CAD build for the part. Positions are in the model's coordinates, mm. A direction names the side the tool comes from. Round coordinates to 2 decimals unless told otherwise and drop trailing zeros. Loops run counter-clockwise (first coordinate to the right, second up) from the corner with the lowest first, then second, coordinate; pieces in that order, holes last. Notation, with made-up numbers: M 29.25,6.5 L 72.25,6.5 A16 ccw 72.25,14.5 Z; hole C 66.5,87 d11. An arc over 180 degrees is marked long. Put each result on its own line as item: value. Start each with the question number.
from build123d import *

# Parameters (mm, degrees)
SKETCH1_W           = 25
SKETCH1_H           = 32
BOSS_EXTRUDE1_DEPTH = 2
SKETCH2_W           = 29
SKETCH2_H           = 36
SKETCH2_W_2         = 25
SKETCH2_H_2         = 32
BOSS_EXTRUDE2_DEPTH = 17
SKETCH3_W           = 18
SKETCH3_H           = 2
CUT_EXTRUDE1_DEPTH  = 2.7
SKETCH4_W           = 8
SKETCH4_H           = 2
CUT_EXTRUDE2_DEPTH  = 1.5
SKETCH7_W           = 1
SKETCH7_H           = 32
BOSS_EXTRUDE3_DEPTH = 15
SKETCH8_W           = 3
SKETCH8_H           = 7.46
CUT_EXTRUDE4_DEPTH  = 6
SKETCH9_W           = 3
SKETCH9_H           = 7.46
CUT_EXTRUDE5_DEPTH  = 6.5
SKETCH10_W          = 29
SKETCH10_H          = 3
BOSS_EXTRUDE4_DEPTH = 5
SKETCH11_W          = 29
SKETCH11_H          = 3
BOSS_EXTRUDE5_DEPTH = 5
SKETCH12_R          = 0.775
CUT_EXTRUDE6_DEPTH  = 4
FILLET1_R           = 5
SKETCH13_R          = 1.275
CUT_EXTRUDE7_DEPTH  = 1
SKETCH14_W          = 5
SKETCH14_H          = 3
BOSS_EXTRUDE6_DEPTH = 5
SKETCH15_W          = 5
SKETCH15_H          = 3
BOSS_EXTRUDE7_DEPTH = 5
SKETCH16_R          = 0.775
CUT_EXTRUDE8_DEPTH  = 5
FILLET2_R           = 2
SKETCH17_R          = 1.275
CUT_EXTRUDE9_DEPTH  = 1
SKETCH18_W          = 1.5
SKETCH18_H          = 5
CUT_EXTRUDE10_DEPTH = 42
SKETCH19_W          = 3
SKETCH19_H          = 3
CUT_EXTRUDE11_DEPTH = 18
SKETCH21_W          = 1.5
SKETCH21_H          = 5
CUT_EXTRUDE12_DEPTH = 2


with BuildPart() as part:
    # Sketch1 → Boss-Extrude1 (new body)
    with BuildSketch(Plane(origin=(0, 0, 0), x_dir=(1, 0, 0), z_dir=(0, 1, 0))):
        with Locations((-1.021545319, 9.369242199)):
            Rectangle(SKETCH1_W, SKETCH1_H)
    extrude(amount=BOSS_EXTRUDE1_DEPTH)

    # Sketch2 → Boss-Extrude2 (add)
    with BuildSketch(Plane(origin=(0, 2, 0), x_dir=(1, 0, 0), z_dir=(0, 1, 0))):
        with Locations((-1.021545319, 9.369242199)):
            Rectangle(SKETCH2_W, SKETCH2_H)
        with Locations((-1.021545319, 9.369242199)):
            Rectangle(SKETCH2_W_2, SKETCH2_H_2, mode=Mode.SUBTRACT)
    extrude(amount=-BOSS_EXTRUDE2_DEPTH)

    # Sketch3 → Cut-Extrude1 (cut)
    with BuildSketch(Plane.XZ.offset(15)):
        with Locations((-4.521545319, -26.369242199)):
            Rectangle(SKETCH3_W, SKETCH3_H)
    extrude(amount=-CUT_EXTRUDE1_DEPTH, mode=Mode.SUBTRACT)

    # Sketch4 → Cut-Extrude2 (cut)
    with BuildSketch(Plane.XZ.offset(15)):
        with Locations((-4.521545319, 7.630757801)):
            Rectangle(SKETCH4_W, SKETCH4_H)
    extrude(amount=-CUT_EXTRUDE2_DEPTH, mode=Mode.SUBTRACT)

    # Sketch7 → Boss-Extrude3 (add)
    with BuildSketch(Plane.XZ):
        with Locations((10.978454681, -9.369242199)):
            Rectangle(SKETCH7_W, SKETCH7_H)
    extrude(amount=BOSS_EXTRUDE3_DEPTH)

    # Sketch8 → Cut-Extrude4 (cut)
    with BuildSketch(Plane.XZ.offset(15)):
        with Locations((11.978454681, 1.400757801)):
            Rectangle(SKETCH8_W, SKETCH8_H)
    extrude(amount=-CUT_EXTRUDE4_DEPTH, mode=Mode.SUBTRACT)

    # Sketch9 → Cut-Extrude5 (cut)
    with BuildSketch(Plane.XZ.offset(15)):
        with Locations((11.978454681, -20.139242199)):
            Rectangle(SKETCH9_W, SKETCH9_H)
    extrude(amount=-CUT_EXTRUDE5_DEPTH, mode=Mode.SUBTRACT)

    # Sketch10 → Boss-Extrude4 (add)
    with BuildSketch(Plane.XY.offset(8.630757801)):
        with Locations((-1.021545319, 0.5)):
            Rectangle(SKETCH10_W, SKETCH10_H)
    extrude(amount=BOSS_EXTRUDE4_DEPTH)

    # Sketch11 → Boss-Extrude5 (add)
    with BuildSketch(Plane(origin=(0, 0, -27.369242199), x_dir=(-1, 0, 0), z_dir=(0, 0, -1))):
        with Locations((1.021545319, 0.5)):
            Rectangle(SKETCH11_W, SKETCH11_H)
    extrude(amount=BOSS_EXTRUDE5_DEPTH)

    # Sketch12 → Cut-Extrude6 (cut, through all)
    with BuildSketch(Plane.XZ.offset(1)):
        with Locations((-10.521545319, 11.130757801)):
            Circle(SKETCH12_R)
        with Locations((8.478454681, 11.130757801)):
            Circle(SKETCH12_R)
        with Locations((8.478454681, -29.869242199)):
            Circle(SKETCH12_R)
        with Locations((-10.521545319, -29.869242199)):
            Circle(SKETCH12_R)
    extrude(amount=-CUT_EXTRUDE6_DEPTH, mode=Mode.SUBTRACT)

    # Fillet1
    fillet1_edges = [part.edges().sort_by_distance(p)[0] for p in [
        (-15.521545319, 0.5, -32.369242199),
        (13.478454681, 0.5, -32.369242199),
        (13.478454681, 0.5, 13.630757801),
        (-15.521545319, 0.5, 13.630757801),
    ]]
    fillet(fillet1_edges, radius=FILLET1_R)

    # Sketch13 → Cut-Extrude7 (cut)
    with BuildSketch(Plane.XZ.offset(1)):
        with Locations((8.478454681, -29.869242199)):
            Circle(SKETCH13_R)
        with Locations((-10.521545319, -29.869242199)):
            Circle(SKETCH13_R)
        with Locations((8.478454681, 11.130757801)):
            Circle(SKETCH13_R)
        with Locations((-10.521545319, 11.130757801)):
            Circle(SKETCH13_R)
    extrude(amount=-CUT_EXTRUDE7_DEPTH, mode=Mode.SUBTRACT)

    # Sketch14 → Boss-Extrude6 (add)
    with BuildSketch(Plane.XY.offset(8.630757801)):
        with Locations((-13.021545319, -13.5)):
            Rectangle(SKETCH14_W, SKETCH14_H)
        with Locations((10.978454681, -13.5)):
            Rectangle(SKETCH14_W, SKETCH14_H)
    extrude(amount=BOSS_EXTRUDE6_DEPTH)

    # Sketch15 → Boss-Extrude7 (add)
    with BuildSketch(Plane(origin=(0, 0, -27.369242199), x_dir=(-1, 0, 0), z_dir=(0, 0, -1))):
        with Locations((-10.978454681, -13.5)):
            Rectangle(SKETCH15_W, SKETCH15_H)
    extrude(amount=BOSS_EXTRUDE7_DEPTH)

    # Sketch16 → Cut-Extrude8 (cut)
    with BuildSketch(Plane.XZ.offset(15)):
        with Locations((10.978454681, 11.130757801)):
            Circle(SKETCH16_R)
        with Locations((-13.021545319, 11.130757801)):
            Circle(SKETCH16_R)
        with Locations((10.978454681, -29.869242199)):
            Circle(SKETCH16_R)
    extrude(amount=-CUT_EXTRUDE8_DEPTH, mode=Mode.SUBTRACT)

    # Fillet2
    fillet2_edges = [part.edges().sort_by_distance(p)[0] for p in [
        (-15.521545319, -13.5, 13.630757801),
        (-10.521545319, -13.5, 13.630757801),
        (13.478454681, -13.5, 13.630757801),
        (8.478454681, -13.5, 13.630757801),
        (13.478454681, -13.5, -32.369242199),
        (8.478454681, -13.5, -32.369242199),
    ]]
    fillet(fillet2_edges, radius=FILLET2_R)

    # Sketch17 → Cut-Extrude9 (cut)
    with BuildSketch(Plane(origin=(0, -12, 0), x_dir=(1, 0, 0), z_dir=(0, 1, 0))):
        with Locations((10.978454681, -11.130757801)):
            Circle(SKETCH17_R)
        with Locations((-13.021545319, -11.130757801)):
            Circle(SKETCH17_R)
        with Locations((10.978454681, 29.869242199)):
            Circle(SKETCH17_R)
    extrude(amount=-CUT_EXTRUDE9_DEPTH, mode=Mode.SUBTRACT)

    # Sketch18 → Cut-Extrude10 (cut, through all)
    with BuildSketch(Plane.XY.offset(8.630757801)):
        with Locations((-1.521545319, -7.596891606)):
            Rectangle(SKETCH18_W, SKETCH18_H)
        with Locations((6.478454681, -7.596891606)):
            Rectangle(SKETCH18_W, SKETCH18_H)
        with Locations((-9.521545319, -7.596891606)):
            Rectangle(SKETCH18_W, SKETCH18_H)
    extrude(amount=-CUT_EXTRUDE10_DEPTH, mode=Mode.SUBTRACT)

    # Sketch19 → Cut-Extrude11 (cut, through all)
    with BuildSketch(Plane(origin=(0, 2, 0), x_dir=(1, 0, 0), z_dir=(0, 1, 0))):
        with Locations((-1.021545319, 21.369242199)):
            Rectangle(SKETCH19_W, SKETCH19_H)
        with Locations((-7.021545319, 21.369242199)):
            Rectangle(SKETCH19_W, SKETCH19_H)
        with Locations((4.978454681, 21.369242199)):
            Rectangle(SKETCH19_W, SKETCH19_H)
        with Locations((-1.021545319, 15.369242199)):
            Rectangle(SKETCH19_W, SKETCH19_H)
        with Locations((4.978454681, 15.369242199)):
            Rectangle(SKETCH19_W, SKETCH19_H)
        with Locations((-1.021545319, 9.369242199)):
            Rectangle(SKETCH19_W, SKETCH19_H)
        with Locations((4.978454681, 9.369242199)):
            Rectangle(SKETCH19_W, SKETCH19_H)
        with Locations((-1.021545319, 3.369242199)):
            Rectangle(SKETCH19_W, SKETCH19_H)
        with Locations((4.978454681, 3.369242199)):
            Rectangle(SKETCH19_W, SKETCH19_H)
        with Locations((-1.021545319, -2.630757801)):
            Rectangle(SKETCH19_W, SKETCH19_H)
        with Locations((4.978454681, -2.630757801)):
            Rectangle(SKETCH19_W, SKETCH19_H)
        with Locations((-7.021545319, 15.369242199)):
            Rectangle(SKETCH19_W, SKETCH19_H)
        with Locations((-7.021545319, 9.369242199)):
            Rectangle(SKETCH19_W, SKETCH19_H)
        with Locations((-7.021545319, 3.369242199)):
            Rectangle(SKETCH19_W, SKETCH19_H)
        with Locations((-7.021545319, -2.630757801)):
            Rectangle(SKETCH19_W, SKETCH19_H)
    extrude(amount=-CUT_EXTRUDE11_DEPTH, mode=Mode.SUBTRACT)

    # Sketch21 → Cut-Extrude12 (cut)
    with BuildSketch(Plane.ZY.offset(15.521545319)):
        with Locations((2.630757801, -7.6)):
            Rectangle(SKETCH21_W, SKETCH21_H)
        with Locations((-3.369242199, -7.6)):
            Rectangle(SKETCH21_W, SKETCH21_H)
        with Locations((-9.369242199, -7.6)):
            Rectangle(SKETCH21_W, SKETCH21_H)
        with Locations((-15.369242199, -7.6)):
            Rectangle(SKETCH21_W, SKETCH21_H)
        with Locations((-21.369242199, -7.6)):
            Rectangle(SKETCH21_W, SKETCH21_H)
    extrude(amount=-CUT_EXTRUDE12_DEPTH, mode=Mode.SUBTRACT)


solid = part.part
(1) Cut at C-C on z = -26.5. List the corners of the cut face in (x, y), and give its area (3 significant figures).
(2) Drill centre lines: line 1 along Z through (x, y) = (-13, -4.75); line 2 along X through (y, z) = (-3.25, -12); line 3 along Z through (x, y) = (10.75, -10). Where is each one in solid material? Low to high.
(3) Flat gauge pins, fed straight in: pin 1 Ø1 at (x, y) = (2, -3) entering from +Z; pin 2 Ø2 at (x, z) = (-4, 7.5) entering from -Y; pin 3 Ø6 at (y, z) = (-11, 0.5) entering from +X; pin 4 Ø1.5 at (x, y) = (12.5, -12) entering from -Z. Where does each tip first touch, or does it go through?
(4) Mould opens along Y. For faces 6 (the flat face through (10, -15, -28)), 7 (the flat face through (-2, -5.097, 8)), 8 (the cylindrical face through (12.05, 0.52, 12.13)) say: +Y half, -Y half, draft (parallel to the pull), parting line (faces both ways), or undercut.
(5) Tool access for faces 1 (the flat face through (9, 0, 12)), 2 (the flat face through (-15, -10.1, 3)), 3 (the flat face through (-8.522, 1, 3)), 4 (the flat face through (-15, -5.1, -21)), 5 (the flat face through (4.478, -14, -26)): list every direction of +Z, -Z, +X, -X, +Y, -Y with a clear straight run to the whole face (end or side of a thin tool).
(6) Cut at B-B on y = -4. List the corners of the cut face in (x, z), and give its area (3 significant figures).
(7) Cut at A-A on x = -6. Count the separate pieces of the cut face and the enclosed holes in it, and give its area (3 significant figures).
Taken from the geometry:
1. outline: M -15.52,-15 L -13.52,-15 L -13.52,-12.3 L 4.48,-12.3 L 4.48,-15 L 13.48,-15 L 13.48,2 L -15.52,2 Z; hole M -10.27,-10.1 L -8.77,-10.1 L -8.77,-5.1 L -10.27,-5.1 Z; hole M -2.27,-10.1 L -0.77,-10.1 L -0.77,-5.1 L -2.27,-5.1 Z; hole M 5.73,-10.1 L 7.23,-10.1 L 7.23,-5.1 L 5.73,-5.1 Z
1. area: 422 mm2
2. line 1: -27.37 to -25.37, 6.63 to 8.63
2. line 2: -15.52 to -13.52, 10.48 to 13.48
2. line 3: -27.37 to -23.87, -16.41 to -2.33, 5.13 to 8.63
3. pin 1: z = 8.63
3. pin 2: y = -13.5
3. pin 3: x = 13.48
3. pin 4: z = -32.35
4. face 6: -Y half
4. face 7: undercut
4. face 8: draft
5. face 1: none
5. face 2: +X, -X
5. face 3: +Y, -Y
5. face 4: -X
5. face 5: -Z, -Y
6. outline: M -15.52,-27.37 L 13.48,-27.37 L 13.48,8.63 L -15.52,8.63 Z; hole M -13.52,-25.37 L 10.48,-25.37 L 10.48,6.63 L -13.52,6.63 Z
6. area: 276 mm2
7. separate pieces: 6
7. enclosed holes: 0
7. area: 124 mm2
